Here's how the part is built. I have some questions about the finished solid (model axes, mm). A direction names the side the tool comes from. Coordinates: 2 decimals unless noted, no trailing zeros. Write each loop counter-clockwise with the first axis right and the second up, starting at its lowest first coordinate (ties: lowest second). Pieces come first, ordered by that corner, then holes. Notation, with made-up numbers: (5, -17.75) -> (18, -17.75) arc R24 ccw to (18, -5.75) -> close; hole circle Ø6 at (-26, 85.5). An arc over 180 degrees is marked (long way). Use a Markdown table: item, result. Add a question column.
Item 1: Imagine slicing it at B-B, the plane x = 72. Write out the boundary of the cut face in (y, z).
Item 2: Will these pins go through, and if not, where does the flat tip stop? pin 1 Ø8 at (x, y) = (25, -2.5) entering from -Z; pin 2 Ø5 at (y, z) = (-6, -18.5) entering from -X; pin 3 Ø12 at (x, y) = (45.5, -12.5) entering from -Z; pin 4 Ø8 at (y, z) = (-16.5, -46.5) entering from -X.
Item 3: If I drill on line 1 along X through (y, z) = (-35, -40); line 2 along Z through (x, y) = (20, -4); line 3 along Y through (x, z) = (17.5, -1), over which ranges is the centre line in solid material (lowest first)? Write a range as from..to.
Item 4: On a 3-axis mill with a long thin cutter (end or side, diameter ignored), from which of +Z, -Z, +X, -X, +Y, -Y can I reach the whole of each face in a straight line? I mean faces 4 (the cylindrical face through (49.76, -36.64, -41.53)), 5 (the cylindrical face through (12.878, 5.037, 0.661)), 6 (the flat face through (0, 0, 0)), 7 (the cylindrical face through (74.785, -37.456, -39.952)). Say none if no direction works.
Item 5: Imagine slicing it at A-A, the plane z = -10. Write out the boundary of the cut face in (x, y).
Item 6: If we mould it in two halves opening along Y, with no side actions, what happens to faces 1 (the cylindrical face through (32.389, -19.314, -41.077)), 2 (the cylindrical face through (36.362, 0.223, -21.341)), 3 (the flat face through (87.686, -34, -46))? For each: pulls with the +Y half, pulls with the -Y half, needs draft (parallel to the pull), parting line crosses it, or undercut.
```python
from build123d import *

# Parameters (mm, degrees)
SKETCH6_R           = 5.08
SKETCH7_R           = 6.858
BOSS_EXTRUDE1_DEPTH = 25.4
FILLET1_R           = 2.54


with BuildPart() as part:
    # Sweep1: sweep along a curve in space
    with BuildLine() as sweep1_path:
        Line((0, 0, 0), (25.4, 0, 0))
        ThreePointArc((25.4, 0, 0), (29.562920183, 0, -1.724337999), (31.287258182, 0, -5.887258182))
        Line((31.287258182, 0, -5.887258182), (31.287258182, 0, -36.367258182))
        ThreePointArc((31.287258182, 0, -36.367258182), (31.287258182, -2.832027095, -43.204376403), (31.287258182, -9.669145315, -46.036403497))
        Line((31.287258182, -9.669145315, -46.036403497), (31.287258182, -28.692102311, -46.036403497))
        ThreePointArc((31.287258182, -28.692102311, -46.036403497), (32.927182179, -32.651229067, -46.036403497), (36.886308936, -34.291153065, -46.036403497))
        Line((36.886308936, -34.291153065, -46.036403497), (62.286308936, -34.291153065, -46.036403497))
    # Sketch6 → Sweep1 (sweep)
    with BuildSketch(Plane(origin=(0, 0, 0), x_dir=(0, 0, -1), z_dir=(1, 0, 0))):
        Circle(SKETCH6_R)
    sweep(path=sweep1_path.line)

    # Sketch7 → Boss-Extrude1 (add)
    with BuildSketch(Plane(origin=(62.286308936, 0, 0), x_dir=(0, 0, -1), z_dir=(1, 0, 0))):
        with Locations(Location((46.036403497, -34.291153065, 0), (0, 0, 270))):
            Circle(SKETCH7_R)
    extrude(amount=BOSS_EXTRUDE1_DEPTH)

    # Fillet1
    # the kernel refuses this fillet: 2.54 mm, written as the material it takes off along each edge
    with BuildSketch(Plane(origin=(62.286308936, -34.291153065, -46.036403497), x_dir=(0, -1, 0), z_dir=(0, 0, 1))) as fillet1_piece_1:
        with BuildLine():
            CenterArc((4.318, 2.423005572), FILLET1_R, 287.457603124, 72.542396876)
            Line((5.08, 0), (5.09524, -0.048460111))
            ThreePointArc((5.09524, -0.048460111), (5.969, -0.0508), (6.858, -0.0508))
            Line((6.858, -0.0508), (6.9088, 0))
            Line((6.9088, 0), (6.9088, 2.423005572))
            Line((6.9088, 2.423005572), (6.858, 2.423005572))
        make_face()
    revolve(axis=Axis((62.286308936, -34.291153065, -46.036403497), (1, 0, 0)), mode=Mode.SUBTRACT)
    with BuildSketch(Plane(origin=(87.686308936, -34.291153065, -46.036403497), x_dir=(0, -1, 0), z_dir=(0, 0, 1))) as fillet1_piece_2:
        with BuildLine():
            CenterArc((6.858 - FILLET1_R, -FILLET1_R), FILLET1_R, 0, 90)
            Line((6.858 - FILLET1_R, 0), (6.858 - FILLET1_R, FILLET1_R * 0.02))
            Line((6.858 - FILLET1_R, FILLET1_R * 0.02), (6.858 + FILLET1_R * 0.02, FILLET1_R * 0.02))
            Line((6.858 + FILLET1_R * 0.02, FILLET1_R * 0.02), (6.858 + FILLET1_R * 0.02, -FILLET1_R))
            Line((6.858 + FILLET1_R * 0.02, -FILLET1_R), (6.858, -FILLET1_R))
        make_face()
    revolve(axis=Axis((87.686308936, -34.291153065, -46.036403497), (1, 0, 0)), mode=Mode.SUBTRACT)


solid = part.part
```
Ans:
| question | item | result |
|---|---|---|
| 1 | outline | circle Ø13.72 at (-34.29, -46.04) |
| 2 | pin 1 | stops at z = -49.26 |
| 2 | pin 2 | stops at x = 27.61 |
| 2 | pin 3 | passes through |
| 2 | pin 4 | stops at x = 26.21 |
| 3 | line 1 | x = 62.88..86.98 |
| 3 | line 2 | z = -3.13..3.13 |
| 3 | line 3 | y = -4.98..4.98 |
| 4 | face 4 | none |
| 4 | face 5 | -X |
| 4 | face 6 | +Z, -Z, -X, +Y, -Y |
| 4 | face 7 | +X |
| 5 | outline | circle Ø10.16 at (31.29, 0) |
| 6 | face 1 | undercut |
| 6 | face 2 | parting line crosses it |
| 6 | face 3 | needs draft |
